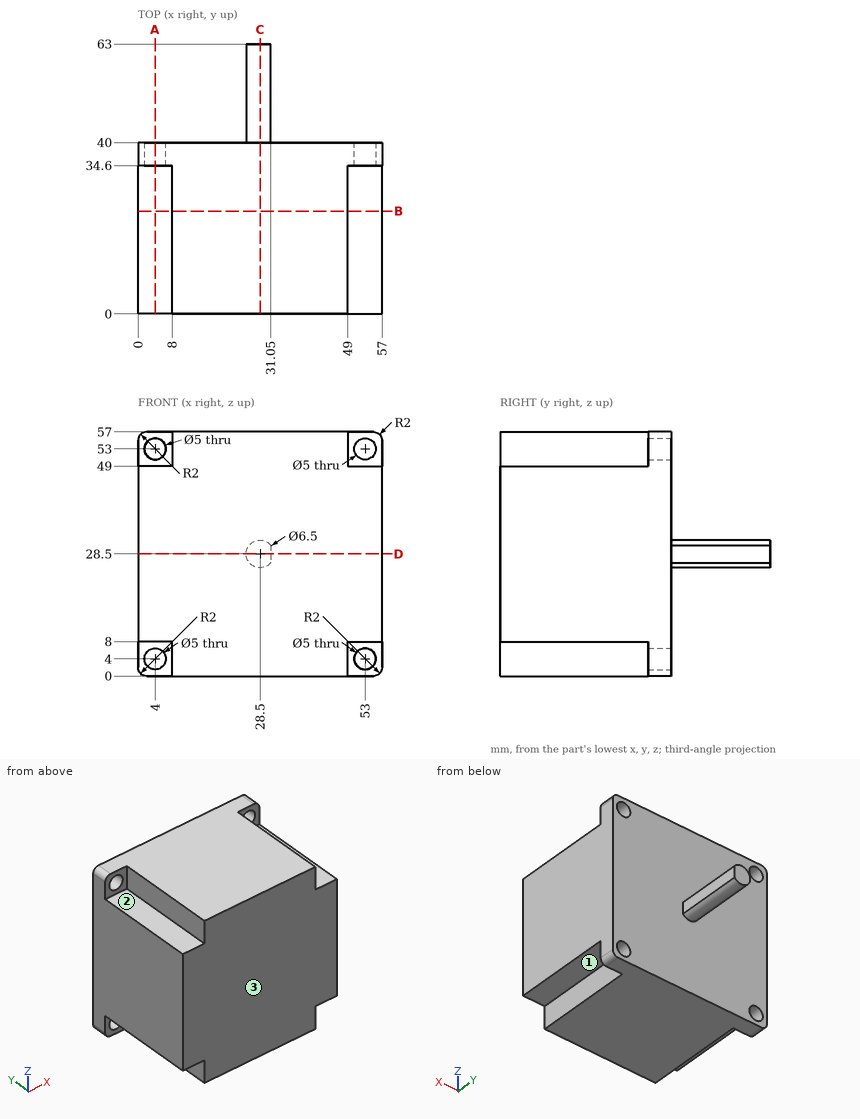
Source: three-view drawing plus pictorial views. Frame: mm from the lowest corner of the part. A direction names the side the tool comes from. Coordinates: 2 decimals unless noted, no trailing zeros. Loops run counter-clockwise (first coordinate to the right, second up) from the corner with the lowest first, then second, coordinate; pieces in that order, holes last. Notation, with made-up numbers: (87, 42.25) -> (140, 42.25) arc R24 cw to (140, 78.25) -> close; hole circle Ø9 at (2.25, 13). An arc over 180 degrees is marked (long way). Answer in a Markdown table with one row per item. Add a question column.
Q1. Section C-C on x = 28.5. Return the cut outline in (y, z), and give its area (3 significant figures).
Q2. Section A-A on x = 4. Return the cut outline in (y, z).
Q3. Section D-D on z = 28.5. Return the cut outline in (x, y), and give its area (3 significant figures).
Q4. Contact query for flat-ended pins moving along their axis: pin 1 Ø8 at (x, z) = (7.5, 17.5) entering from -Y; pin 2 Ø1 at (x, z) = (41, 39) entering from +Y; pin 3 Ø4 at (y, z) = (21.5, 52) entering from +X; pin 4 Ø1 at (y, z) = (51.5, 27) entering from +X. Output: stop coordinate, or through.
Q5. Section B-B on y = 24. Return the cut outline in (x, z), and give its area (3 significant figures).
Q6. Reachability of the marked faces 1, 2 and 3 from +Z, -Z, +X, -X, +Y, -Y: full face, straight path, thin tool, end or side. Return the list, or none.
Q7. Ray query, line 1 along X through (y, z) = (36.95, 53); line 2 along Y through (x, z) = (54.5, 42). Return the intervals inside material, ascending.
Computed values:
| question | item | result |
|---|---|---|
| 1 | outline | (0, 0) -> (40, 0) -> (40, 25.25) -> (63, 25.25) -> (63, 31.75) -> (40, 31.75) -> (40, 57) -> (0, 57) -> close |
| 1 | area | 2,430 mm^2 |
| 2 | outline | (0, 8) -> (34.6, 8) -> (34.6, 6.5) -> (40, 6.5) -> (40, 50.5) -> (34.6, 50.5) -> (34.6, 49) -> (0, 49) -> close; (34.6, 0) -> (40, 0) -> (40, 1.5) -> (34.6, 1.5) -> close; (34.6, 55.5) -> (40, 55.5) -> (40, 57) -> (34.6, 57) -> close |
| 3 | outline | (0, 0) -> (57, 0) -> (57, 40) -> (31.05, 40) -> (31.05, 63) -> (25.25, 63) -> (25.25, 40) -> (0, 40) -> close |
| 3 | area | 2,410 mm^2 |
| 4 | pin 1 | stops at y = 0 |
| 4 | pin 2 | stops at y = 40 |
| 4 | pin 3 | stops at x = 49 |
| 4 | pin 4 | stops at x = 31.05 |
| 5 | outline | (0, 8) -> (8, 8) -> (8, 0) -> (49, 0) -> (49, 8) -> (57, 8) -> (57, 49) -> (49, 49) -> (49, 57) -> (8, 57) -> (8, 49) -> (0, 49) -> close |
| 5 | area | 2,990 mm^2 |
| 6 | face 1 | -Z, +X, -Y |
| 6 | face 2 | +Z, -X, -Y |
| 6 | face 3 | +Z, -Z, +X, -X, -Y |
| 7 | line 1 | x = 0 to 1.5, 6.5 to 50.5, 55.5 to 57 |
| 7 | line 2 | y = 0 to 40 |
